Can you work these out from the model? Positions are in its coordinate system, mm. Face numbers are marked on the shaded views. A direction names the side the tool comes from. Give positions to 0.01 mm unless a question says otherwise; leave off trailing zeros. Loops run counter-clockwise (first coordinate to the right, second up) from the corner with the lowest first, then second, coordinate; pieces in that order, holes last. Notation, with made-up numbers: (36.5, 12.25) -> (80.5, 12.25) arc R33 ccw to (80.5, 49.25) -> close; hole circle Ø8 at (53.5, 24.5). An arc over 180 degrees is marked (long way). Return JSON: item names as keys, results as strings. Group by question number.
Q1. Suppose I cut it at B-B, the plane z = 4. Please give me the cut outline in (x, y), and give its area (3 significant figures).
Q2. Suppose I cut it at A-A, the plane y = 16.75. Please give me the cut outline in (x, z), and give its area (3 significant figures).
Q3. Will this pin go through, and if not, where does the flat tip stop? pin 1 (1 mm diameter, centred on x = 17, z = -11, fed in from +Y).
Q4. Which directions (+Z, -Z, +X, -X, +Y, -Y) give clear straight access to the entire face, cutting with the end or side of a thin tool? Please do the marked faces 4 and 5.
Q5. Suppose I cut it at D-D, the plane z = -33. Please give me the cut outline in (x, y), and give its area (3 significant figures).
Q6. Thinking about a two-plate mould opening in X: for the marked faces 1, 2 and 3, which applies, pulls with the +X half, pulls with the -X half, needs draft (parallel to the pull), parting line crosses it, or undercut?
Q7. Suppose I cut it at C-C, the plane x = -29.5. Please give me the cut outline in (y, z).
Q8. I need wall thicknesses on line 1 along X through (y, z) = (14.25, -3); line 2 along Z through (x, y) = (-6.5, 6.5); line 3 along Y through (x, z) = (34.5, -20). Which ranges of each line are inside material? Lowest first, please. Write a range as [from, to].
```python
from build123d import *

# Parameters (mm, degrees)
SKETCH1_W           = 101.6
SKETCH1_H           = 76.2
SKETCH1_R           = 1.524
BOSS_EXTRUDE1_DEPTH = 3
SKETCH1_3_R         = 1.524
BOSS_EXTRUDE2_DEPTH = 25
SKETCH1_4_W         = 105.264465986
SKETCH1_4_H         = 80.768961322
SKETCH1_4_W_2       = 101.6
SKETCH1_4_H_2       = 76.2
BOSS_EXTRUDE3_DEPTH = 20


with BuildPart() as part:
    # Sketch1 → Boss-Extrude1 (new body)
    with BuildSketch(Plane(origin=(0, 0, 0), x_dir=(1, 0, 0), z_dir=(0, 1, 0))):
        Rectangle(SKETCH1_W, SKETCH1_H)
        with Locations(Location((-42.370602661, -32.936523162, 0), (0, 0, 270))):
            Circle(SKETCH1_R, mode=Mode.SUBTRACT)
        with Locations(Location((42.205092494, -33.267543495, 0), (0, 0, 270))):
            Circle(SKETCH1_R, mode=Mode.SUBTRACT)
        with Locations(Location((42.205092494, 32.605502829, 0), (0, 0, 270))):
            Circle(SKETCH1_R, mode=Mode.SUBTRACT)
        with Locations(Location((-41.91, 33.147, 0), (0, 0, 270))):
            Circle(SKETCH1_R, mode=Mode.SUBTRACT)
    extrude(amount=BOSS_EXTRUDE1_DEPTH)

    # Sketch1_3 → Boss-Extrude2 (add)
    with BuildSketch(Plane(origin=(0, 0, 0), x_dir=(1, 0, 0), z_dir=(0, 1, 0))):
        with Locations(Location((-41.91, 33.147, 0), (0, 0, 270))):
            Circle(SKETCH1_3_R)
        with Locations(Location((42.205092494, 32.605502829, 0), (0, 0, 270))):
            Circle(SKETCH1_3_R)
        with Locations(Location((42.205092494, -33.267543495, 0), (0, 0, 270))):
            Circle(SKETCH1_3_R)
        with Locations(Location((-42.370602661, -32.936523162, 0), (0, 0, 270))):
            Circle(SKETCH1_3_R)
    extrude(amount=BOSS_EXTRUDE2_DEPTH)

    # Sketch1_4 → Boss-Extrude3 (add)
    with BuildSketch(Plane(origin=(0, 0, 0), x_dir=(1, 0, 0), z_dir=(0, 1, 0))):
        Rectangle(SKETCH1_4_W, SKETCH1_4_H)
        Rectangle(SKETCH1_4_W_2, SKETCH1_4_H_2, mode=Mode.SUBTRACT)
    extrude(amount=BOSS_EXTRUDE3_DEPTH)


solid = part.part
```
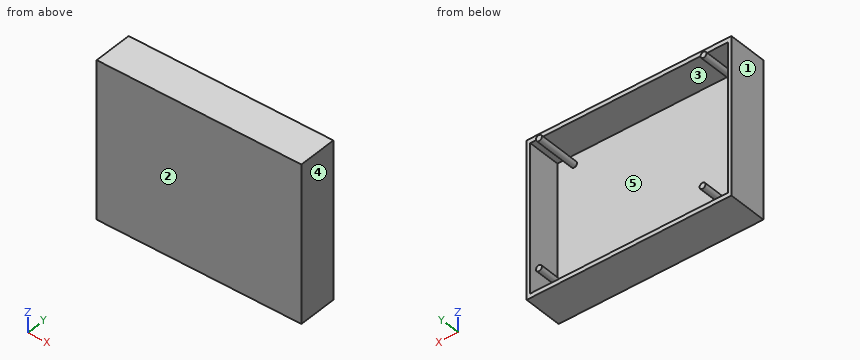
Ans:
{
 "1": {"outline": "(-52.63, 0) -> (52.63, 0) -> (52.63, 20) -> (50.8, 20) -> (50.8, 3) -> (-50.8, 3) -> (-50.8, 20) -> (-52.63, 20) -> close", "area": "378 mm^2"},
 "2": {"outline": "(-52.63, -40.38) -> (52.63, -40.38) -> (52.63, 40.38) -> (-52.63, 40.38) -> close; circle Ø3.05 at (-42.37, 32.94); circle Ø3.05 at (-41.91, -33.15); circle Ø3.05 at (42.21, -32.61); circle Ø3.05 at (42.21, 33.27); hole (-50.8, -38.1) -> (50.8, -38.1) -> (50.8, 38.1) -> (-50.8, 38.1) -> close", "area": "789 mm^2"},
 "3": {"pin 1": "stops at y = 3"},
 "4": {"face 4": "+Z, -Z, +X, +Y, -Y", "face 5": "+Y"},
 "5": {"outline": "(-52.63, 0) -> (52.63, 0) -> (52.63, 20) -> (50.8, 20) -> (50.8, 3) -> (43.68, 3) -> (43.68, 25) -> (40.73, 25) -> (40.73, 3) -> (-40.39, 3) -> (-40.39, 25) -> (-43.43, 25) -> (-43.43, 3) -> (-50.8, 3) -> (-50.8, 20) -> (-52.63, 20) -> close", "area": "510 mm^2"},
 "6": {"face 1": "pulls with the -X half", "face 2": "needs draft", "face 3": "undercut"},
 "7": {"outline": "(0, -40.38) -> (20, -40.38) -> (20, -38.1) -> (3, -38.1) -> (3, 38.1) -> (20, 38.1) -> (20, 40.38) -> (0, 40.38) -> close"},
 "8": {"line 1": "x = [-52.63, -50.8], [50.8, 52.63]", "line 2": "z = [-40.38, -38.1], [38.1, 40.38]", "line 3": "y = [0, 3]"}
}
